The drawing under review shows one solid part. Ordinate dimensions are in mm from its lowest x, y, z. A direction names the side the tool comes from. Give positions to 0.01 mm unless a question says otherwise; leave off trailing zeros. Loops run counter-clockwise (first coordinate to the right, second up) from the corner with the lowest first, then second, coordinate; pieces in that order, holes last. Notation, with made-up numbers: (54, -3.75) -> (72, -3.75) arc R32 ccw to (72, 31.25) -> close; hole circle Ø1 at (-2, 15.5). An arc over 180 degrees is marked (long way). Answer in a Markdown table with one row per item. Add a question column.
(1) Draft analysis for pull direction X (two halves, no side actions). For the marked faces 1, 2 and 3, state which applies: +X half, -X half, draft (parallel to the pull), parting line (faces both ways), or undercut.
(2) For pin 1 (2 mm diameter, centred on y = 2.5, z = 9, fed in from -X); pin 2 (10 mm diameter, centred on x = 28.5, z = 3.5, fed in from -Y); pin 3 (5 mm diameter, centred on x = 11.25, z = 5, fed in from +Y); pin 4 (4 mm diameter, centred on y = 5, z = 18, fed in from +X), all flat-tipped, find the tip position at first contact; note any pin that passes through.
(3) Consider section A-A on x = 37. Write out the cut boundary in (y, z), then the cut area to 3 significant figures.
(4) Consider section B-B on z = 6.25. Write out the cut boundary in (x, y), then the cut area to 3 significant figures.
(5) For line 1 (X direction, y = 5, z = 2.7); line 2 (X direction, y = 8.25, z = 3.25); line 3 (X direction, y = 5, z = 3.5), list the stretches that pass through material, from the lowest coordinate up.
(6) Consider section D-D on z = 4. Write out the cut boundary in (x, y) (1 decimal), then the cut area to 3 significant figures.
(7) Consider section C-C on y = 9.25. Count the separate pieces of the cut face and the enclosed holes in it, then the cut area to 3 significant figures.
(8) For the marked faces 4, 5, 6 and 7, list the 3-axis set-ups (+Z, -Z, +X, -X, +Y, -Y) from which the entire face can be reached by the end or side of a thin tool; tool diameter is ignored.
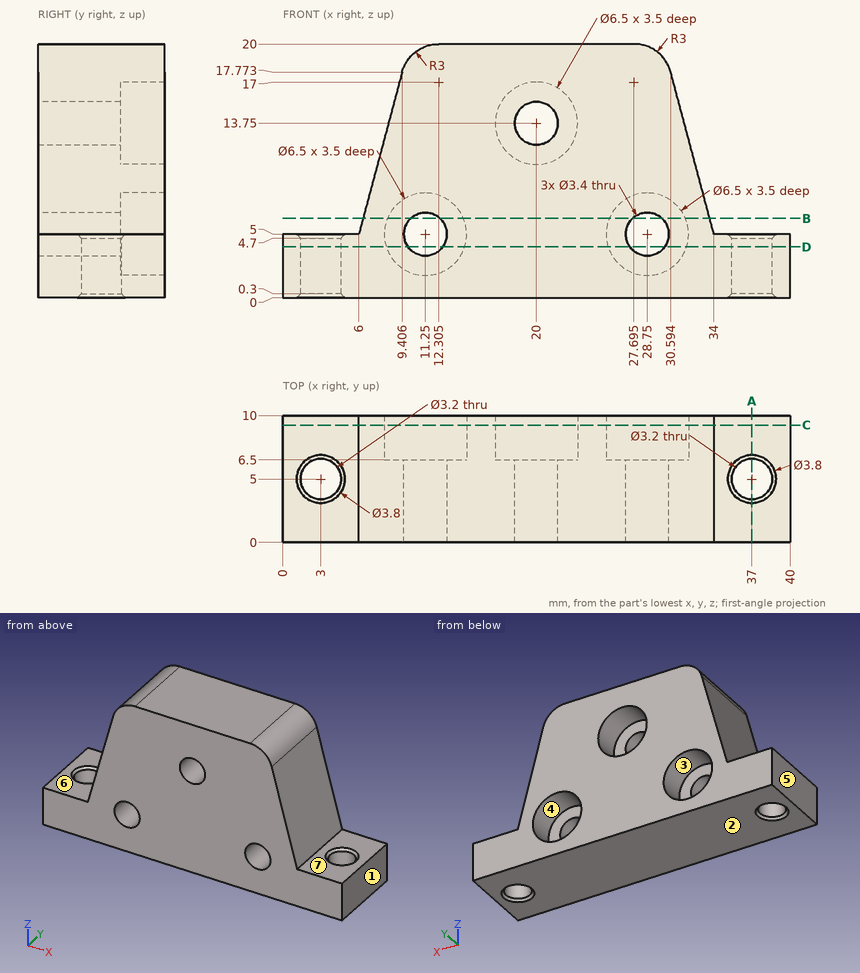
Values follow:
| question | item | result |
|---|---|---|
| 1 | face 1 | +X half |
| 1 | face 2 | draft |
| 1 | face 3 | undercut |
| 2 | pin 1 | x = 6.8 |
| 2 | pin 2 | y = 0 |
| 2 | pin 3 | y = 6.5 |
| 2 | pin 4 | x = 31.07 |
| 3 | outline | (0, 0) -> (3.1, 0) -> (3.4, 0.3) -> (3.4, 4.7) -> (3.1, 5) -> (0, 5) -> close; (6.6, 0.3) -> (6.9, 0) -> (10, 0) -> (10, 5) -> (6.9, 5) -> (6.6, 4.7) -> close |
| 3 | area | 33.8 mm2 |
| 4 | outline | (6.33, 0) -> (10.1, 0) -> (10.1, 6.5) -> (8.25, 6.5) -> (8.25, 10) -> (6.33, 10) -> close; (12.4, 0) -> (27.6, 0) -> (27.6, 6.5) -> (25.75, 6.5) -> (25.75, 10) -> (14.25, 10) -> (14.25, 6.5) -> (12.4, 6.5) -> close; (29.9, 0) -> (33.67, 0) -> (33.67, 10) -> (31.75, 10) -> (31.75, 6.5) -> (29.9, 6.5) -> close |
| 4 | area | 201 mm2 |
| 5 | line 1 | 0 to 1.4, 4.6 to 35.4, 38.6 to 40 |
| 5 | line 2 | 0 to 8.51, 13.99 to 26.01, 31.49 to 40 |
| 5 | line 3 | 0 to 1.4, 4.6 to 10.45, 12.05 to 27.95, 29.55 to 35.4, 38.6 to 40 |
| 6 | outline | (0, 0) -> (9.9, 0) -> (9.9, 6.5) -> (8.2, 6.5) -> (8.2, 10) -> (0, 10) -> close; (12.6, 0) -> (27.4, 0) -> (27.4, 6.5) -> (25.7, 6.5) -> (25.7, 10) -> (14.3, 10) -> (14.3, 6.5) -> (12.6, 6.5) -> close; (30.1, 0) -> (40, 0) -> (40, 10) -> (31.8, 10) -> (31.8, 6.5) -> (30.1, 6.5) -> close; hole circle Ø3.2 at (3, 5); hole circle Ø3.2 at (37, 5) |
| 6 | area | 305 mm2 |
| 7 | separate pieces | 1 |
| 7 | enclosed holes | 3 |
| 7 | area | 458 mm2 |
| 8 | face 4 | +Y |
| 8 | face 5 | +Z, -Z, -X, +Y, -Y |
| 8 | face 6 | +Z, -X, +Y, -Y |
| 8 | face 7 | +Z, +X, +Y, -Y |
